Build history of the part. All positions in model axes, mm. Coordinates: 2 decimals unless noted, no trailing zeros. Order: outer loops, then holes, each group sorted by start corner. A loop starts at its lowest first (then second) coordinate and runs counter-clockwise, first axis right, second up. Notation, with made-up numbers: (63.5, 80.25) - (78.5, 80.25) arc R9 ccw to (78.5, 94.25) - close; hole circle Ø8 at (-12, 35). An arc over 180 degrees is marked (long way). Return JSON: item names as keys, results as strings.
from build123d import *

# Parameters (mm, degrees)
SKETCH1_W           = 150
SKETCH1_H           = 150
BOSS_EXTRUDE1_DEPTH = 59
SKETCH2_W           = 111.9
SKETCH2_H           = 111.9
CUT_EXTRUDE1_DEPTH  = 60
SKETCH9_R           = 1.4
CUT_EXTRUDE4_DEPTH  = 20
CIRPATTERN1_COUNT   = 3
CIRPATTERN1_ANGLE   = 180
SKETCH10_W          = 111.9
SKETCH10_H          = 105.448295943
CUT_EXTRUDE6_DEPTH  = 60
SKETCH11_W          = 19.05
SKETCH11_H          = 19.05
CUT_EXTRUDE7_DEPTH  = 60


with BuildPart() as part:
    # Sketch1 → Boss-Extrude1 (new body)
    with BuildSketch(Plane(origin=(0, 0, 0), x_dir=(1, 0, 0), z_dir=(0, 1, 0))):
        Rectangle(SKETCH1_W, SKETCH1_H)
    extrude(amount=-BOSS_EXTRUDE1_DEPTH)

    # Sketch2 → Cut-Extrude1 (cut, through all)
    with BuildSketch(Plane(origin=(0, 0, 0), x_dir=(1, 0, 0), z_dir=(0, 1, 0))):
        Rectangle(SKETCH2_W, SKETCH2_H)
    extrude(amount=-CUT_EXTRUDE1_DEPTH, mode=Mode.SUBTRACT)

    # Sketch9 → Cut-Extrude4 (cut)
    with BuildSketch(Plane.ZY.offset(75)):
        with Locations((-6.1, -7.25)):
            Circle(SKETCH9_R)
        with Locations((6.1, -7.25)):
            Circle(SKETCH9_R)
        with Locations((6.1, -15.25)):
            Circle(SKETCH9_R)
        with Locations((-6.1, -15.25)):
            Circle(SKETCH9_R)
    cut_extrude4 = extrude(amount=-CUT_EXTRUDE4_DEPTH, mode=Mode.SUBTRACT)

    # CirPattern1: Cut-Extrude4 ×3 about axis
    cirpattern1_axis = Axis((0, 0, 0), (0, 1, 0))
    for i in range(1, CIRPATTERN1_COUNT):
        add(cut_extrude4.rotate(cirpattern1_axis, i * CIRPATTERN1_ANGLE / (CIRPATTERN1_COUNT - 1)), mode=Mode.SUBTRACT)

    # Sketch10 → Cut-Extrude6 (cut, through all)
    with BuildSketch(Plane(origin=(0, 0, 0), x_dir=(1, 0, 0), z_dir=(0, 1, 0))):
        with Locations((0, 108.674147972)):
            Rectangle(SKETCH10_W, SKETCH10_H)
    extrude(amount=-CUT_EXTRUDE6_DEPTH, mode=Mode.SUBTRACT)

    # Sketch11 → Cut-Extrude7 (cut, through all)
    with BuildSketch(Plane(origin=(0, 0, 0), x_dir=(1, 0, 0), z_dir=(0, 1, 0))):
        Polygon((75, 75), (-55.95, 75), (-55.95, -55.95), (-55.95, -75), (75, -75), align=None)
        with Locations((-65.475, -65.475)):
            Rectangle(SKETCH11_W, SKETCH11_H)
    extrude(amount=-CUT_EXTRUDE7_DEPTH, mode=Mode.SUBTRACT)


solid = part.part
1. Mould opens along Y. For faces 1 (the flat face through (-55.95, -29, -9)), 2 (the flat face through (-66, -59, -10)), 3 (the cylindrical face through (-65.6, -14.1, 6.9)) say: pulls with the +Y half, pulls with the -Y half, needs draft (parallel to the pull), parting line crosses it, or undercut.
Check values:
{"face 1": "needs draft", "face 2": "pulls with the -Y half", "face 3": "undercut"}
2. Cut at A-A on z = 6.1. Give the cut face in (x, y), plus the area to 3 significant figures.
Check values:
{"outline": "(-75, -59) - (-55.95, -59) - (-55.95, -16.65) - (-75, -16.65) - close; (-75, -13.85) - (-55.95, -13.85) - (-55.95, -8.65) - (-75, -8.65) - close; (-75, -5.85) - (-55.95, -5.85) - (-55.95, 0) - (-75, 0) - close", "area": "1,020 mm²"}
3. Probe L1, parallel to Y at x = -69, z = -6.1; L2, parallel to Y at x = -72.25, z = 5.5; L3, parallel to Z at x = -66, y = -6. List the from-to ranges inside material, lowest first.
Check values:
{"L1": "-59 to -16.65, -13.85 to -8.65, -5.85 to 0", "L2": "-59 to -16.51, -13.99 to -8.51, -5.99 to 0", "L3": "-75 to -6.73, -5.47 to 5.47, 6.73 to 55.95"}
4. Drop flat-ended pins along their axis: pin 1 (2.5 mm diameter, centred on y = -7.25, z = -6.1, fed in from -X); pin 2 (4.5 mm diameter, centred on y = -15.25, z = 6.1, fed in from -X). Give the stop position or say it passes through.
Check values:
{"pin 1": "through", "pin 2": "x = -75"}
5. Cut at B-B on y = -7.25. Give the cut face in (x, z), plus the area to 3 significant figures.
Check values:
{"outline": "(-75, -75) - (-55.95, -75) - (-55.95, -7.5) - (-75, -7.5) - close; (-75, -4.7) - (-55.95, -4.7) - (-55.95, 4.7) - (-75, 4.7) - close; (-75, 7.5) - (-55.95, 7.5) - (-55.95, 55.95) - (-75, 55.95) - close", "area": "2,390 mm²"}
